```python
from build123d import *

# Parameters (mm, degrees)
CUT_EXTRUDE1_DEPTH = 1.5


with BuildPart() as part:
    # Sketch1 → Revolve1 (revolve)
    with BuildSketch(Plane(origin=(0, 0, 0), x_dir=(1, 0, 0), z_dir=(0, 1, 0)), mode=Mode.PRIVATE) as revolve1_sk:
        with BuildLine():
            Line((1.5, 0), (1.5, 10))
            Line((1.5, 10), (2.85, 10))
            add(Edge.make_bspline(
                [(1.5, 11.65), (2.631595647, 10.927172538), (2.85, 10)],
                knots=[0, 0, 0, 0.488855094, 0.488855094, 0.488855094], degree=2))
            Line((1.5, 11.65), (0, 11.65))
            Line((0, 11.65), (0, 0))
            Line((0, 0), (1.5, 0))
        make_face()
    revolve(revolve1_sk.sketch.rotate(Axis((0, 0, -11.65), (0, 0, 1)), 180), axis=Axis((0, 0, -11.65), (0, 0, 1)))

    # Sketch2 → Cut-Extrude1 (cut)
    with BuildSketch(Plane(origin=(0, 0, -11.65), x_dir=(-1, 0, 0), z_dir=(0, 0, -1))):
        Polygon((0.576895528, 1.000262407), (-0.577804891, 0.999737386), (-1.154700419, -0.000525021), (-0.576895528, -1.000262407), (0.577804891, -0.999737386), (1.154700419, 0.000525021), align=None)
    extrude(amount=-CUT_EXTRUDE1_DEPTH, mode=Mode.SUBTRACT)


solid = part.part
```
Can you work these out from the model? Positions are in its coordinate system, mm. A direction names the side the tool comes from. Give positions to 0.01 mm unless a question says otherwise; leave off trailing zeros. Loops run counter-clockwise (first coordinate to the right, second up) from the corner with the lowest first, then second, coordinate; pieces in that order, holes last. Notation, with made-up numbers: M 61.25,75.25 L 110.25,75.25 A22 cw 110.25,85.25 Z; hole C -28,62 d7. An arc over 180 degrees is marked long. Use CSV: the item, a comma, the result in double quotes. Start each with the question number.
1. For P1, Ø1.5, axis at x = 1.5, z = -10.5, coming from the -Y side; P2, Ø1.6, axis at x = -0.5, y = 0, coming from the -Z side; P3, Ø2, axis at y = 1.5, z = -6.5, coming from the -X side, each with a flat end and sliding along its axis, tell me the tip position at first contact or that it passes through.
2. If we mould it in two halves opening along X, with no side actions, what happens to faces 3 (the face through (-0.87, 0.49, -10.91)), 4 (the face through (-1.43, -0.45, -5.07)), 5 (the face through (0, 0, 0))? For each: released by +X, released by -X, zero draft, split by the parting line, or undercut.
3. If I drill on L1, parallel to Z at x = 0.35, y = 0.05; L2, parallel to X at y = -1, z = -6; L3, parallel to X at y = 1.25, z = -4.25, over which ranges is the centre line in solid material (lowest first)?
4. Imagine slicing it at A-A, the plane z = -2.25. Write out the boundary of the cut face in (x, y).
5. On a 3-axis mill with a long thin cutter (end or side, diameter ignored), from which of +Z, -Z, +X, -X, +Y, -Y can I reach the whole of each face in a straight line? I mean faces 1 (the face through (0.87, -0.49, -10.91)), 2 (the face through (1.2, 1.2, -10)). Say none if no direction works.
Response values:
1,P1,"y = -2.69"
1,P2,"z = -11.65"
1,P3,"x = -1.41"
2,face 3,"undercut"
2,face 4,"split by the parting line"
2,face 5,"zero draft"
3,L1,"-10.15 to 0"
3,L2,"-1.12 to 1.12"
3,L3,"-0.83 to 0.83"
4,outline,"C 0,0 d3"
5,face 1,"-Z"
5,face 2,"+Z"
